The listing builds one solid part. Answer for the finished solid, in the listing's coordinates (mm). A direction names the side the tool comes from. Give positions to 0.01 mm unless a question says otherwise; leave off trailing zeros. Loops run counter-clockwise (first coordinate to the right, second up) from the corner with the lowest first, then second, coordinate; pieces in that order, holes last.
Item 1: The mould has two halves that part along X. Classify faces 1 (the face through (-0.081, -144.762, 36.164)), 2 (the face through (-50.045, -125, -1)), 3 (the face through (38.02, -187.48, 3.81)): pulls with the +X half, pulls with the -X half, needs draft (parallel to the pull), parting line crosses it, or undercut.
Item 2: Consider line 1 along X through (y, z) = (-169, -8); line 2 along Z through (x, y) = (22, -80); line 3 along Y through (x, z) = (16, 9.5). Determine where each line is inside the solid, lowest interval first.
Item 3: Section B-B, the plane x = -17 is taken. Give the vertices of the cut face in (y, z).
Item 4: Section C-C, the plane y = -146 is taken. Give the vertices of the cut face in (x, z).
Item 5: Section A-A, the plane z = 0 is taken. Give the vertices of the cut face in (x, y), and give its area (3 significant figures).
Item 6: A tool of negligible diameter and unlimited length cuts with its end or side. For faces 4 (the face through (-38.136, -250.181, 39.786)), 5 (the face through (-0.081, -144.762, -36.164)), 6 (the face through (-1, -152.4, 0)), from which of +Z, -Z, +X, -X, +Y, -Y can it reach the whole face along a straight path? Write none if from no direction.
Item 7: Each of these flat-tipped pins is pushed along its axis until it touches: pin 1 Ø20.5 at (y, z) = (-199.6, 0) entering from -X; pin 2 Ø11 at (x, z) = (2.5, 8.5) entering from -Y. Where does it stop, or does it pass through?
Item 8: Section D-D, the plane z = 15.5 is taken. Give the vertices of the cut face in (x, y).
from build123d import *

# Parameters (mm, degrees)
F0_W     = 100.0908872011
F0_H     = 86.8150984859
F1_DEPTH = 152.4
F2_W     = 23.4895850481
F2_H     = 86.8150984859
F2_W_2   = 0.6694942713
F2_W_3   = 23.7127671899
F3_DEPTH = 101.6
F4_R     = 12.7
F6_D     = 25.4
F7_R     = 25.4


with BuildPart() as f1:
    # F0 (on Front) → F1 (new body)
    with BuildSketch(Plane.XZ):
        Rectangle(F0_W, F0_H)
    extrude(amount=F1_DEPTH)

    # F2 (on face) → F3 (join)
    with BuildSketch(Plane.XZ.offset(152.4)):
        with Locations((-38.3006510765, 0)):
            Rectangle(F2_W, F2_H)
        Polygon((25.6631821394, 43.9454764128), (25.6631821394, 43.4075492429), (26.3326764107, 43.4075492429), (50.0454436006, 43.4075492429), (50.0454436006, 43.9454764128), align=None)
        with Locations((25.997929275, 0)):
            Rectangle(F2_W_2, F2_H)
        with Locations((38.1890600056, 0)):
            Rectangle(F2_W_3, F2_H)
    extrude(amount=F3_DEPTH)

    # F4
    f4_edges = [f1.edges().sort_by_distance(p)[0] for p in [
        (-38.300651, -254, -43.407549),
        (37.854313, -254, -43.407549),
        (37.854313, -254, 43.945476),
        (-38.300651, -254, 43.407549),
    ]]
    fillet(f4_edges, radius=F4_R)

    # F6 (through all)
    with Locations(Plane(origin=(-50.0454436006, 0, 0), x_dir=(0, -1, 0), z_dir=(-1, 0, 0))):
        with Locations((199.5964795351, 0)):
            Hole(F6_D / 2)

    # F7
    f7_edges = [f1.edges().sort_by_distance(p)[0] for p in [
        (-0.446338, -152.4, -43.407549),
        (-0.446338, -152.4, 43.407549),
    ]]
    fillet(f7_edges, radius=F7_R)


solid = f1.part
Worked answers:
1. face 1: undercut
1. face 2: pulls with the -X half
1. face 3: needs draft
2. line 1: x = -50.05 to -26.56, 25.66 to 50.05
2. line 2: z = -43.41 to 43.41
2. line 3: y = -152.4 to 0
3. outline: (-152.4, -18.01) arc R25.4 ccw to (-127, -43.41) - (0, -43.41) - (0, 43.41) - (-127, 43.41) arc R25.4 ccw to (-152.4, 18.01) - close
4. outline: (-50.05, -43.41) - (-26.56, -43.41) - (-26.56, -34.86) - (25.66, -34.86) - (25.66, -43.41) - (50.05, -43.41) - (50.05, 43.41) - (25.66, 43.41) - (25.66, 34.86) - (-26.56, 34.86) - (-26.56, 43.41) - (-50.05, 43.41) - close
5. outline: (-50.05, -254) - (-26.56, -254) - (-26.56, -212.3) - (-50.05, -212.3) - close; (-50.05, -186.9) - (-26.56, -186.9) - (-26.56, -152.4) - (25.66, -152.4) - (25.66, -186.9) - (50.05, -186.9) - (50.05, 0) - (-50.05, 0) - close; (25.66, -254) - (50.05, -254) - (50.05, -212.3) - (25.66, -212.3) - close
5. area: 18,900 mm2
6. face 4: +Z, -X, -Y
6. face 5: -Z, -Y
6. face 6: +Z, -Z, -Y
7. pin 1: passes through
7. pin 2: stops at y = -152.4
8. outline: (-50.05, -254) - (-26.56, -254) - (-26.56, -152.4) - (25.66, -152.4) - (25.66, -254) - (50.05, -254) - (50.05, 0) - (-50.05, 0) - close
